Design review of the part built by this model. Coordinates are the model's own, in mm. Face numbers are marked on the shaded views. A direction names the side the tool comes from. Round coordinates to 2 decimals unless told otherwise and drop trailing zeros. Order: outer loops, then holes, each group sorted by start corner. A loop starts at its lowest first (then second) coordinate and runs counter-clockwise, first axis right, second up. Notation, with made-up numbers: (-6.75, 39.5) - (8.25, 39.5) arc R20 ccw to (8.25, 48.5) - close; hole circle Ø5 at (81.5, 47.25). An arc over 180 degrees is marked (long way). Answer as a JSON object with one key per item and string values. Group by question number.
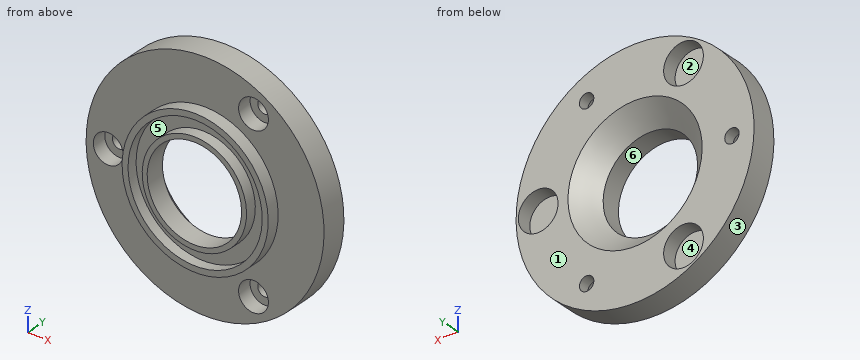
Autodesk Inventor part; units mm, degrees
ref_plane "YZ Plane" through (0, 0, 0) normal (1, 0, 0) x (0, 1, 0)
ref_plane "XZ Plane" through (0, 0, 0) normal (0, 1, 0) x (-1, 0, 0)
ref_plane "XY Plane" through (0, 0, 0) normal (0, 0, 1) x (1, 0, 0)
ref_plane "Arbeitsebene1" through (20.8918, -10.7106, -13.7095) normal (1, 0, 0) x (0, 1, 0)
sketch "Skizze1" plane through (20.8918, -10.7106, -13.7095) normal (1, 0, 0) x (0, 1, 0)
  circle A0 centre (0.052, 12) radius 1.5 construction
  line L0 (13.1827, 0) -> (-4.1221, 0)
  line L1 (-1.248, 10.5) -> (1.552, 10.5)
  line L2 (1.552, 10.5) -> (1.552, 13.5)
  line L3 (1.552, 13.5) -> (-1.048, 13.5)
  line L4 (1.552, 23.9428) -> (6.752, 23.9428)
  line L5 (6.752, 23.9428) -> (6.752, 13.5)
  line L6 (2.752, 9.5) -> (-1.248, 9.5)
  line L7 (-1.248, 9.5) -> (-1.248, 10.5)
  line L8 (6.752, 13.5) -> (2.752, 9.5)
  line L9 (-1.048, 13.5) -> (-1.048, 14.7029)
  line L10 (1.05, -14.9922) -> (1.05, 14.9922) construction
  line L11 (-1.4, -14.9922) -> (-1.4, 14.9922) construction
  line L12 (1.05, 14.9029) -> (-1.4, 14.9029) construction
  line L13 (-1.048, 14.7029) -> (1.552, 14.7029)
  line L14 (1.552, 14.7029) -> (1.552, 23.9428)
  line L15 (-2.25, 23.9428) -> (1.15, 23.9428)
  point P0 (10.7106, 13.7095)
  point P1 (6.752, 9.5)
  point P2 (-1.048, 14.9029)
  dimension "d0" = 3
  dimension "d1" = 12
  dimension "d4" = 4
  dimension "d5" = 4
  dimension "d6" = 1
  dimension "d7" = 1.3
  dimension "d8" = 2.6
  dimension "d10" = 4
  dimension "d11" = 0.2
  dimension "d20" = 0
revolve "Umdrehung1" add sketch "Skizze1" angle 360 about axis through (20.8918, 2.4721, -13.7095) along (0, -1, 0)
sketch "Skizze2" plane through (20.8918, -9.1586, -13.7095) normal (0, -1, 0) x (1, 0, 0)
  circle A0 centre (9.7461, 16.8807) radius 4
  circle A1 centre (-19.4922, 0) radius 4
  circle A2 centre (9.7461, -16.8807) radius 4
  point P0 (-20.8918, 13.7095)
hole "Bohrung1" at (30.6379, -9.1586, 3.1712) at (30.6379, -9.1586, -30.5903) at (1.3996, -9.1586, -13.7095) direction (0, 1, 0) diameter 2.9 depth 12 tip angle 118 counterbore diameter 6 counterbore depth 3
sketch "Skizze3" plane through (20.8918, -3.9586, -13.7095) normal (0, 1, 0) x (1, 0, 0)
  circle A0 centre (0, 0) radius 13.5
  circle A1 centre (9.7461, -16.8807) radius 1.45
  circle A2 centre (0, 0) radius 19.4922 construction
  line L0 (-9.7461, -16.8807) -> (-9.7461, 16.8807) construction
  line L1 (-9.7461, 16.8807) -> (19.4922, 0) construction
  line L2 (19.4922, 0) -> (-9.7461, -16.8807) construction
  circle A3 centre (-9.7461, -16.8807) radius 4
  circle A4 centre (-9.7461, 16.8807) radius 4
  circle A5 centre (19.4922, 0) radius 4
  point P0 (-20.8918, -13.7095)
  dimension "d21" = 8
  dimension "d22" = 8
  dimension "d23" = 8
extrude "Extrusion1" cut sketch "Skizze3" against normal blind 3 contours A3 | A4 | A5
sketch "Skizze4" plane through (20.8918, -9.1586, -13.7095) normal (0, -1, 0) x (1, 0, 0)
  circle A0 centre (0, 0) radius 13.5
  circle A1 centre (0, 0) radius 10.5
  point P0 (-20.8918, 13.7095)
extrude "Extrusion2" add sketch "Skizze4" along normal blind 0.5
properties part number "01_SMLM_Holder_Base"
1. To check wall thickness, follow line 1 (Z direction, x = 23, y = -11.5); line 2 (X direction, y = -5.25, z = -30); line 3 (Y direction, x = 33, z = -22.5). State the ranges of each line that lie inside material, in increasing order. Write a range as from..to.
2. Take a section at B-B, the plane y = -5.25. Give the boundary of the cut face in (x, z), then the cut area to 3 significant figures.
3. Take a section at C-C, the plane y = -10.75. Give the boundary of the cut face in (x, z).
4. Take a section at A-A, the plane x = 42. Give the boundary of the cut face in (y, z).
5. Tool access review of the marked faces 4, 5 and 6: name each direction out of +Z, -Z, +X, -X, +Y, -Y from which nothing blocks a thin tool from reaching the whole face with its end or side.
6. Clearance check with flat-ended pins moving along their axes: P1, Ø4.5, axis at x = 30.64, z = 3.17, coming from the -Y side; P2, Ø7, axis at x = 40.38, z = -13.71, coming from the -Y side; P3, Ø8, axis at x = 14, z = -13.5, coming from the +Y side; P4, Ø16, axis at x = 20.89, z = -13.71, coming from the -Y side. State where each tip first meets the part, or that it passes through.
7. Mouldability with a two-part tool opening along X and no side actions: class the marked faces 1, 2 and 3 as pulls with the +X half, pulls with the -X half, needs draft (parallel to the pull), parting line crosses it, or undercut.
Response values:
{
 "1": {"line 1": "-28.26..-27.04, -24..-22.97, -4.45..-3.42, -0.38..0.84", "line 2": "3.35..7.19, 15.1..29.31, 31.96..38.44", "line 3": "-9.16..-3.96"},
 "2": {"outline": "circle Ø47.89 at (20.89, -13.71); hole circle Ø2.9 at (1.4, -13.71); hole circle Ø8 at (11.15, -30.59); hole circle Ø8 at (11.15, 3.17); hole circle Ø24.42 at (20.89, -13.71); hole circle Ø2.9 at (30.64, -30.59); hole circle Ø2.9 at (30.64, 3.17); hole circle Ø8 at (40.38, -13.71)", "area": "1,160 mm2"},
 "3": {"outline": "circle Ø29.41 at (20.89, -13.71); circle Ø21 at (20.89, -13.71); hole circle Ø27 at (20.89, -13.71); hole circle Ø19 at (20.89, -13.71)"},
 "4": {"outline": "(-9.16, -25.01) - (-3.96, -25.01) - (-3.96, -17.37) - (-6.96, -17.37) - (-6.96, -10.05) - (-3.96, -10.05) - (-3.96, -2.41) - (-9.16, -2.41) - close"},
 "5": {"face 4": "+Y", "face 5": "-Y", "face 6": "+Y, -Y"},
 "6": {"P1": "y = -6.16", "P2": "y = -9.16", "P3": "y = -6.56", "P4": "through"},
 "7": {"face 1": "needs draft", "face 2": "undercut", "face 3": "parting line crosses it"}
}
